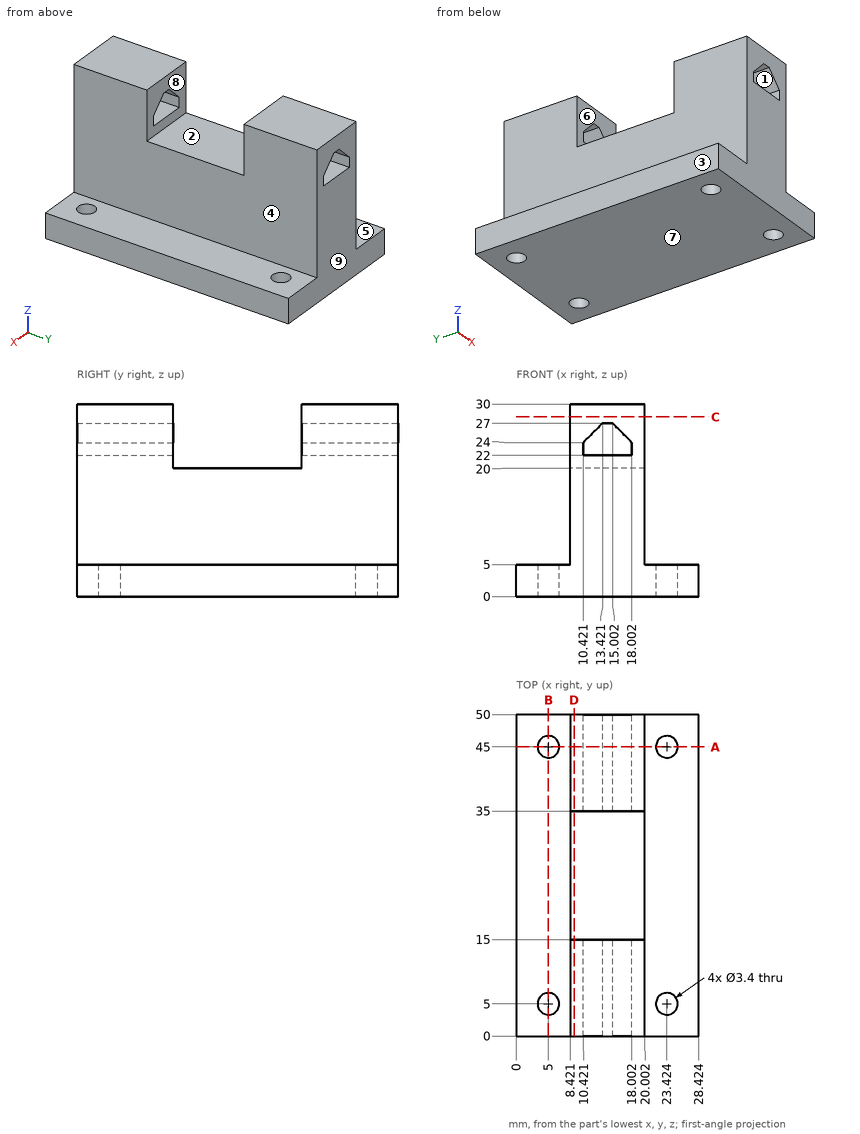
Input: dimensioned drawing with shaded views. Units: mm. Origin: part minimum x, y, z. A direction names the side the tool comes from. Give positions to 0.01 mm unless a question says otherwise; leave off trailing zeros. Write each loop counter-clockwise with the first axis right and the second up, starting at its lowest first coordinate (ties: lowest second). Pieces come first, ordered by that corner, then holes. Notation, with made-up numbers: (-31.5, -39) - (-6.5, -39) arc R32 ccw to (-6.5, -3) - close; hole circle Ø3 at (-5.75, -23.75). An arc over 180 degrees is marked (long way). One line per item, written item: value. Start each with the question number.
Q1. First-contact query: pin 1 Ø3.5 at (x, y) = (17, 26) entering from +Z; pin 2 Ø0.6 at (y, z) = (43, 23) entering from -X; pin 3 Ø2 at (x, y) = (7, 31.5) entering from +Z; pin 4 Ø1 at (x, z) = (20, 13) entering from -Y. Flat tips, straight axial feed; report the tip coordinate or a pass-through.
Q2. Draft query along Y for the marked faces 6, 7, 8 and 9. Return one class per face: +Y half, -Y half, draft (parallel to the pull), parting line (faces both ways), or undercut.
Q3. Section query A-A, the plane y = 45. Return the cut outline in (x, z).
Q4. Section query D-D, the plane x = 9. Return the cut outline in (y, z).
Q5. Set-up query: the marked faces 1, 2, 3, 4 and 5. Return all of +Z, -Z, +X, -X, +Y, -Y with unobstructed straight access to the full face (end or side cutting, diameter ignored); none if empty.
Q6. Section query C-C, the plane z = 28. Return the cut outline in (x, y).
Q7. Section query B-B, the plane x = 5. Return the cut outline in (y, z), then the cut area to 3 significant figures.
Q8. Material intervals for probe 1 along X at (y, z) = (5, 2.5); probe 2 along Y at (x, z) = (5, 3); probe 3 along Z at (x, y) = (14.25, 46), sorted ascending. Write a range as from..to.
Answer:
1. pin 1: stops at z = 20
1. pin 2: stops at x = 8.42
1. pin 3: stops at z = 5
1. pin 4: stops at y = 0
2. face 6: undercut
2. face 7: draft
2. face 8: undercut
2. face 9: +Y half
3. outline: (0, 0) - (3.3, 0) - (3.3, 5) - (0, 5) - close; (6.7, 0) - (21.72, 0) - (21.72, 5) - (20, 5) - (20, 30) - (8.42, 30) - (8.42, 5) - (6.7, 5) - close; (25.12, 0) - (28.42, 0) - (28.42, 5) - (25.12, 5) - close; hole (10.42, 22) - (18, 22) - (18, 24) - (15, 27) - (13.42, 27) - (10.42, 24) - close
4. outline: (0, 0) - (50, 0) - (50, 30) - (35, 30) - (35, 20) - (15, 20) - (15, 30) - (0, 30) - close
5. face 1: +Y, -Y
5. face 2: +Z, +X, -X
5. face 3: +Z, -Z, -X, +Y, -Y
5. face 4: +Z, +X, +Y, -Y
5. face 5: +Z, -X, +Y, -Y
6. outline: (8.42, 0) - (20, 0) - (20, 15) - (8.42, 15) - close; (8.42, 35) - (20, 35) - (20, 50) - (8.42, 50) - close
7. outline: (0, 0) - (3.3, 0) - (3.3, 5) - (0, 5) - close; (6.7, 0) - (43.3, 0) - (43.3, 5) - (6.7, 5) - close; (46.7, 0) - (50, 0) - (50, 5) - (46.7, 5) - close
7. area: 216 mm2
8. probe 1: x = 0..3.3, 6.7..21.72, 25.12..28.42
8. probe 2: y = 0..3.3, 6.7..43.3, 46.7..50
8. probe 3: z = 0..22, 27..30
